Could you check a few things on this model? Use its own coordinates, in mm. A direction names the side the tool comes from. Round coordinates to 2 decimals unless told otherwise and drop trailing zeros. Write each loop counter-clockwise with the first axis right and the second up, starting at its lowest first coordinate (ties: lowest second). Pieces come first, ordered by that corner, then holes.
```python
from build123d import *

# Parameters (mm, degrees)
BOSS_EXTRUDE1_DEPTH = 10
FILLET1_R           = 6
FILLET2_R           = 2
FILLET3_R           = 2
SKETCH2_R           = 4
CUT_EXTRUDE1_DEPTH  = 34.113449774


with BuildPart() as part:
    # Sketch1 → Boss-Extrude1 (new body)
    with BuildSketch(Plane.XY):
        with BuildLine():
            Line((-27.171188048, -9.347902097), (-27.171188048, -6.180932375))
            ThreePointArc((-27.171188048, -6.180932375), (-27.771188048, -4.347902097), (-27.171188048, -2.514871819))
            Line((-27.171188048, -2.514871819), (-27.171188048, 4.485128181))
            Line((-27.171188048, 4.485128181), (-22.171188048, 4.485128181))
            Line((-22.171188048, 4.485128181), (-22.171188048, -2.514871819))
            ThreePointArc((-22.171188048, -2.514871819), (-21.725004076, -3.38353702), (-21.571188048, -4.347902097))
            ThreePointArc((-21.571188048, -4.347902097), (-21.725004076, -5.312267173), (-22.171188048, -6.180932375))
            Line((-22.171188048, -6.180932375), (-22.171188048, -9.347902097))
            Line((-22.171188048, -9.347902097), (-19.171188048, -9.347902097))
            Line((-19.171188048, -9.347902097), (-19.171188048, 7.485128181))
            Line((-19.171188048, 7.485128181), (-30.171188048, 7.485128181))
            Line((-30.171188048, 7.485128181), (-30.171188048, -9.347902097))
            Line((-30.171188048, -9.347902097), (-27.171188048, -9.347902097))
        make_face()
    extrude(amount=BOSS_EXTRUDE1_DEPTH)

    # Fillet1
    # the kernel refuses this fillet: 6 mm, written as the material it takes off along each edge
    with BuildSketch(Plane(origin=(-19.171188048, 7.485128181, -15), x_dir=(-1, 0, 0), z_dir=(0, 0, 1))) as fillet1_piece_1:
        with BuildLine():
            CenterArc((FILLET1_R, FILLET1_R), FILLET1_R, 180, 90)
            Line((0, FILLET1_R), (0, 0))
            Line((0, 0), (FILLET1_R, 0))
        make_face()
    extrude(amount=40, mode=Mode.SUBTRACT)
    with BuildSketch(Plane(origin=(-30.171188048, 7.485128181, -15), x_dir=(1, 0, 0), z_dir=(0, 0, 1))) as fillet1_piece_2:
        with BuildLine():
            CenterArc((FILLET1_R, -FILLET1_R), FILLET1_R, 90, 90)
            Line((0, -FILLET1_R), (0, 0))
            Line((0, 0), (FILLET1_R, 0))
        make_face()
    extrude(amount=40, mode=Mode.SUBTRACT)

    # Fillet2
    # the kernel refuses this fillet: 2 mm, written as the material it takes off along each edge
    with BuildSketch(Plane(origin=(-19.171188048, -9.347902097, -5), x_dir=(0, 1, 0), z_dir=(0, 0, 1)), Plane(origin=(-22.171188048, -9.347902097, -5), x_dir=(1, 0, 0), z_dir=(0, 0, 1)), Plane(origin=(-30.171188048, -9.347902097, -5), x_dir=(1, 0, 0), z_dir=(0, 0, 1))) as fillet2_piece_1:
        with BuildLine():
            CenterArc((FILLET2_R, FILLET2_R), FILLET2_R, 180, 90)
            Line((0, FILLET2_R), (0, 0))
            Line((0, 0), (FILLET2_R, 0))
        make_face()
    extrude(amount=20, mode=Mode.SUBTRACT)
    with BuildSketch(Plane(origin=(-27.171188048, -9.347902097, -5), x_dir=(-1, 0, 0), z_dir=(0, 0, 1))) as fillet2_piece_2:
        with BuildLine():
            CenterArc((FILLET2_R, -FILLET2_R), FILLET2_R, 90, 90)
            Line((0, -FILLET2_R), (0, 0))
            Line((0, 0), (FILLET2_R, 0))
        make_face()
    extrude(amount=20, mode=Mode.SUBTRACT)

    # Fillet3
    fillet3_edges = [part.edges().sort_by_distance(p)[0] for p in [
        (-22.171188048, 4.485128181, 5),
        (-27.171188048, 4.485128181, 5),
    ]]
    fillet(fillet3_edges, radius=FILLET3_R)

    # Sketch2 → Cut-Extrude1 (cut, through all)
    with BuildSketch(Plane.XY.offset(10)):
        with Locations((-24.671188048, -4.347902097)):
            Circle(SKETCH2_R)
    extrude(amount=-CUT_EXTRUDE1_DEPTH, mode=Mode.SUBTRACT)


solid = part.part
```
Q1. We'd pull the mould along X, two halves only. Please class faces 4 (the cylindrical face through (-26.57, 3.915, 5.07)), 5 (the cylindrical face through (-21.726, -8.606, 4.93)), 6 (the flat face through (-28, 1, 10)), 7 (the cylindrical face through (-20.71, 5.5, 4.93)): pulls with the +X half, pulls with the -X half, needs draft (parallel to the pull), parting line crosses it, or undercut.
Q2. Imagine slicing it at A-A, the plane y = -1. Write out the boundary of the cut face in (x, z), then the cut area to 3 significant figures.
Q3. If I drill on L1, parallel to X at y = 1, z = 3.75; L2, parallel to X at y = -4.5, z = 6; L3, parallel to Y at x = -22, z = 6.75, over which ranges is the centre line in solid material (lowest first)?
Q4. Imagine slicing it at C-C, the plane z = 6.75. Write out the boundary of the cut face in (x, y), then the cut area to 3 significant figures.
Q5. Imagine slicing it at B-B, the plane x = -27.75. Write out the boundary of the cut face in (y, z).
Q6. I'm going to push flat-ended pins straight in: pin 1 Ø6 at (y, z) = (5, 7) entering from +X; pin 2 Ø1.5 at (x, z) = (-25, 4) entering from -Y; pin 3 Ø2 at (x, y) = (-25, 5) entering from -Z. Where does each tip first touch, or does it pass through?
Q7. Imagine slicing it at D-D, the plane x = -26.25. Write out the boundary of the cut face in (y, z).
Q8. On a 3-axis mill with a long thin cutter (end or side, diameter ignored), from which of +Z, -Z, +X, -X, +Y, -Y can I reach the whole of each face in a straight line? I mean faces 1 (the flat face through (-27.171, 1, 5)), 2 (the cylindrical face through (-28.67, -4.3, 5.07)), 3 (the cylindrical face through (-19.601, -8.587, 4.93)). Say none if no direction works.
Results found:
1. face 4: undercut
1. face 5: undercut
1. face 6: needs draft
1. face 7: pulls with the +X half
2. outline: (-30.17, 0) - (-27.17, 0) - (-27.17, 10) - (-30.17, 10) - close; (-22.17, 0) - (-19.17, 0) - (-19.17, 10) - (-22.17, 10) - close
2. area: 60.0 mm2
3. L1: x = -30.17 to -27.17, -22.17 to -19.17
3. L2: x = -30.17 to -28.67, -20.67 to -19.17
3. L3: y = -8.16 to -7.33, -1.37 to 6.58
4. outline: (-30.17, -7.35) arc R2 ccw to (-28.67, -9.28) arc R2 ccw to (-27.17, -7.47) arc R4 cw to (-27.17, -1.23) - (-27.17, 2.49) arc R2 cw to (-25.17, 4.49) - (-24.17, 4.49) arc R2 cw to (-22.17, 2.49) - (-22.17, -1.23) arc R4 cw to (-22.17, -7.47) arc R2 ccw to (-20.67, -9.28) arc R2 ccw to (-19.17, -7.35) - (-19.17, 1.49) arc R6 ccw to (-24.67, 7.46) arc R6 ccw to (-30.17, 1.49) - close
4. area: 85.8 mm2
5. outline: (-8.76, 0) - (-6.9, 0) - (-6.9, 10) - (-8.76, 10) - close; (-1.79, 0) - (6.3, 0) - (6.3, 10) - (-1.79, 10) - close
6. pin 1: stops at x = -19.19
6. pin 2: stops at y = 4.4
6. pin 3: stops at z = 0
7. outline: (4.17, 0) - (7.11, 0) - (7.11, 10) - (4.17, 10) - close
8. face 1: +Z, -Z, -Y
8. face 2: +Z, -Z
8. face 3: +Z, -Z, +X, -Y
